Model file for the job. Use its own axes, mm. Coordinates: 2 decimals unless noted, no trailing zeros. Write each loop counter-clockwise with the first axis right and the second up, starting at its lowest first coordinate (ties: lowest second). Pieces come first, ordered by that corner, then holes. Notation, with made-up numbers: M 65,76.25 L 104,76.25 A15 cw 104,102.25 Z; hole C 4,-3.75 d6. An arc over 180 degrees is marked long. Use CSV: the item, a comma, the result in double quotes. Start each with the question number.
from build123d import *

# Parameters (mm, degrees)
EXTRUDE_1_DEPTH     = 6
SKETCH_2_R          = 13
SKETCH_2_R_2        = 1.6
CUT_EXTRUDE_1_DEPTH = 6
FILLET_1_R          = 10
SKETCH_3_R          = 1.6
CUT_EXTRUDE_2_DEPTH = 6


with BuildPart() as part:
    # 草图1 → 凸台-拉伸1 (new body)
    with BuildSketch(Plane(origin=(0, 0, 0), x_dir=(1, 0, 0), z_dir=(0, 1, 0))):
        with BuildLine():
            Line((23.77389059, 45), (23.77389059, -45))
            Line((23.77389059, -45), (14.77389059, -45))
            Line((14.77389059, -45), (-23.77389059, -27.249829127))
            ThreePointArc((-23.77389059, -27.249829127), (-41.22610941, 0), (-23.77389059, 27.249829127))
            Line((-23.77389059, 27.249829127), (14.77389059, 45))
            Line((14.77389059, 45), (23.77389059, 45))
        make_face()
    extrude(amount=EXTRUDE_1_DEPTH)

    # 草图2 → 切除-拉伸1 (cut)
    with BuildSketch(Plane(origin=(0, 6, 0), x_dir=(1, 0, 0), z_dir=(0, 1, 0))):
        with Locations(Location((-11.22610941, 0, 0), (0, 0, 270))):
            Circle(SKETCH_2_R)
        with Locations(Location((-31.22610941, 0, 0), (0, 0, 270))):
            Circle(SKETCH_2_R_2)
        with Locations(Location((-1.22610941, -17.320508076, 0), (0, 0, 270))):
            Circle(SKETCH_2_R_2)
        with Locations(Location((-1.22610941, 17.320508076, 0), (0, 0, 270))):
            Circle(SKETCH_2_R_2)
    extrude(amount=-CUT_EXTRUDE_1_DEPTH, mode=Mode.SUBTRACT)

    # 圆角1
    fillet_1_edges = [part.edges().sort_by_distance(p)[0] for p in [
        (14.77389059, 3, -45),
        (14.77389059, 3, 45),
    ]]
    fillet(fillet_1_edges, radius=FILLET_1_R)

    # 草图3 → 切除-拉伸2 (cut)
    with BuildSketch(Plane(origin=(0, 6, 0), x_dir=(1, 0, 0), z_dir=(0, 1, 0))):
        with Locations(Location((12.77389059, 35, 0), (0, 0, 270))):
            Circle(SKETCH_3_R)
        with Locations(Location((12.77389059, -35, 0), (0, 0, 270))):
            Circle(SKETCH_3_R)
    extrude(amount=-CUT_EXTRUDE_2_DEPTH, mode=Mode.SUBTRACT)


solid = part.part
1) Band-saw the part on D-D on x = -26. List the corners of the cut face in (y, z), then the cut area to 3 significant figures.
2) Drop flat-ended pins along their axis: P1, Ø1.5, axis at y = 4.5, z = 2, coming from the -X side; P2, Ø1, axis at y = 2, z = 22, coming from the -X side; P3, Ø5, axis at x = -1.23, z = 17.32, coming from the -Y side; P4, Ø1.5, axis at x = 7, y = 2, coming from the -Z side. Give the stop position or say it passes through.
3) Band-saw the part on C-C on y = 5. List the corners of the cut face in (x, z), then the cut area to 3 significant figures.
4) Wall check: L1, parallel to Z at x = 13.5, y = 2.85; L2, parallel to Z at x = -15, y = 0.4; L3, parallel to X at y = 1.4, z = -5. Give the ranges that are in metal, low to high. Write a range as [from, to].
5) Band-saw the part on A-A on z = 0. List the corners of the cut face in (x, y).
6) Band-saw the part on B-B on z = 35. List the corners of the cut face in (x, y), then the cut area to 3 significant figures.
7) Two-plate mould, pull along Z, no slides. Class faces 1 (the face through (20, 3, -45)), 2 (the face through (-32.788, 3.042, -0.347)), 3 (the face through (-5.24, 2.958, 35.784)), 4 (the face through (-0.75, 3.04, 18.85)): pulls with the +Z half, pulls with the -Z half, needs draft (parallel to the pull), parting line crosses it, or undercut.
Findings below:
1,outline,"M 0,-26.11 L 6,-26.11 L 6,26.11 L 0,26.11 Z"
1,area,"313 mm2"
2,P1,"stops at x = -41.2"
2,P2,"stops at x = -32.15"
2,P3,"stops at y = 0"
2,P4,"stops at z = -41.77"
3,outline,"M -23.77,-27.25 L 12.78,-44.08 A10 ccw 16.97,-45 L 23.77,-45 L 23.77,45 L 16.97,45 A10 ccw 12.78,44.08 L -23.77,27.25 A30 ccw Z; hole C -31.23,0 d3.2; hole C -11.23,0 d26; hole C -1.23,-17.32 d3.2; hole C -1.23,17.32 d3.2; hole C 12.77,-35 d3.2; hole C 12.77,35 d3.2"
3,area,"3,710 mm2"
4,L1,"z = [-44.38, -36.43], [-33.57, 33.57], [36.43, 44.38]"
4,L2,"z = [-31.29, -12.44], [12.44, 31.29]"
4,L3,"x = [-40.81, -23.23], [0.77, 23.77]"
5,outline,"M -41.23,0 L -32.83,0 L -32.83,6 L -41.23,6 Z; M -29.63,0 L -24.23,0 L -24.23,6 L -29.63,6 Z; M 1.77,0 L 23.77,0 L 23.77,6 L 1.77,6 Z"
6,outline,"M -6.94,0 L 11.17,0 L 11.17,6 L -6.94,6 Z; M 14.37,0 L 23.77,0 L 23.77,6 L 14.37,6 Z"
6,area,"165 mm2"
7,face 1,"pulls with the -Z half"
7,face 2,"undercut"
7,face 3,"pulls with the +Z half"
7,face 4,"undercut"
